Job drawing, mm, ordinate dimensions from the low corner. One solid piece. Round coordinates to 2 decimals unless told otherwise and drop trailing zeros. Loops run counter-clockwise (first coordinate to the right, second up) from the corner with the lowest first, then second, coordinate; pieces in that order, holes last. Notation, with made-up numbers: M 43,88.25 L 74,88.25 A34 ccw 74,124.25 Z; hole C 38.25,42.5 d9. An arc over 180 degrees is marked long. Use one line per item in the form item = value.
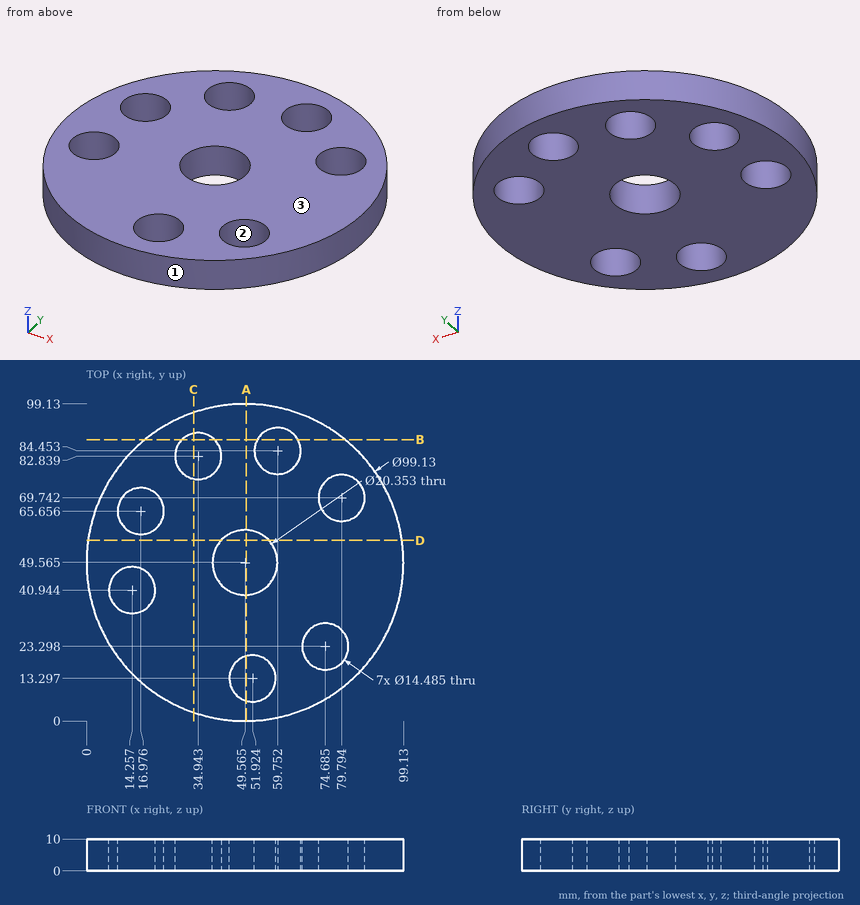
1. Cut at B-B on y = 88. Write the cut outline in (x, z) (1 decimal).
Completed:
outline = M 18.3,0 L 29.9,0 L 29.9,10 L 18.3,10 Z; M 40,0 L 53.4,0 L 53.4,10 L 40,10 Z; M 66.1,0 L 80.9,0 L 80.9,10 L 66.1,10 Z
2. Pull direction X, two halves, no side cores. Call the marked faces 1, 2 and 3: +X half, -X half, draft (parallel to the pull), parting line (faces both ways), or undercut.
Completed:
face_1 = parting line
face_2 = undercut
face_3 = draft
3. Cut at D-D on y = 56.5. Write the cut outline in (x, z).
Completed:
outline = M 0.49,0 L 42.12,0 L 42.12,10 L 0.49,10 Z; M 57.01,0 L 98.64,0 L 98.64,10 L 57.01,10 Z
4. Cut at C-C on x = 33.5. Write the cut outline in (y, z) (1 decimal), and give its area (3 significant figures).
Completed:
outline = M 2.7,0 L 75.7,0 L 75.7,10 L 2.7,10 Z; M 89.9,0 L 96.5,0 L 96.5,10 L 89.9,10 Z
area = 796 mm2
5. Cut at A-A on x = 50. Write the cut outline in (y, z) (1 decimal), and give its area (3 significant figures).
Completed:
outline = M 0,0 L 6.3,0 L 6.3,10 L 0,10 Z; M 20.3,0 L 39.4,0 L 39.4,10 L 20.3,10 Z; M 59.7,0 L 99.1,0 L 99.1,10 L 59.7,10 Z
area = 648 mm2
6. Drop flat-ended pins along their axis: P1, Ø1.5, axis at y = 78, z = 4, coming from the -X side; P2, Ø11.5, axis at x = 79.79, y = 69.74, coming from the +Z side; P3, Ø16.5, axis at x = 14.26, y = 40.94, coming from the +Z side; P4, Ø4, axis at x = 67, z = 6.5, coming from the +Y side (1 decimal). Give the stop position or say it passes through.
Completed:
P1 = 8.45
P2 = through
P3 = 10
P4 = 96.7
7. Probe line 1 along Y through (x, z) = (54.5, 9.25) (1 decimal); line 2 along X through (y, z) = (47.5, 2.75) (1 decimal); line 3 along X through (y, z) = (41.5, 0.75) (1 decimal). List the from-to ranges inside material, lowest first. Write a range as from..to.
Completed:
line_1 = 0.2..6.5, 20.1..40.7, 58.5..79.5, 89.4..98.9
line_2 = 0..11.2, 17.3..39.6, 59.5..99.1
line_3 = 0.7..7, 21.5..43.4, 55.8..98.5
